Read the model definition and answer for the solid it produces. Units are mm, in the model's axes. Face numbers are marked on the shaded views. A direction names the side the tool comes from. Coordinates: 2 decimals unless noted, no trailing zeros. Loops run counter-clockwise (first coordinate to the right, second up) from the corner with the lowest first, then second, coordinate; pieces in that order, holes last. Notation, with made-up numbers: (29.5, -14) - (59.5, -14) arc R20 cw to (59.5, 22) - close; hole circle Ø7 at (26.5, 50.5). An arc over 180 degrees is marked (long way). Use one line per item in the form item = value. Start each with the question number.
1) Which of the six approach directions +Z, -Z, +X, -X, +Y, -Y give full straight-line access (tool end or side, diameter ignored) to the marked faces 1, 2, 3 and 4?
2) A cutting plane is placed at B-B (y = -1). Give the vertices of the cut face in (x, z), and give its area (3 significant figures).
3) A cutting plane is placed at D-D (x = 12.5). Give the vertices of the cut face in (y, z) (3 decimals).
4) Each of these flat-tipped pins is pushed along its axis until it touches: P1, Ø16.5, axis at x = 0, z = 0, coming from the +Y side; P2, Ø5, axis at x = 14, y = -8, coming from the +Z side; P3, Ø8, axis at x = -0.5, y = 24, coming from the -Z side; P4, Ø5, axis at x = 8, z = 12.5, coming from the +Y side. Where does it stop, or does it pass through?
5) A cutting plane is placed at A-A (x = 0). Give the vertices of the cut face in (y, z).
6) A cutting plane is placed at C-C (z = 3). Give the vertices of the cut face in (x, y).
7) The mould has two halves that part along Z. Classify the marked faces 5, 6 and 7: released by +Z, released by -Z, zero draft, split by the parting line, or undercut.
8) Consider line 1 (X direction, y = -19, z = 0); line 2 (Z direction, x = 0, y = 7); line 3 (Y direction, x = -8.5, z = 8.5). Determine where each line is inside the solid, lowest interval first.
from build123d import *

# Parameters (mm, degrees)
F0_R     = 15.24
F0_R_2   = 10.414
F1_DEPTH = 26.67
F2_DEPTH = 38.1
F4_DEPTH = 26.67
F3_R     = 10.414
F5_DEPTH = 19.05
F7_DEPTH = 4.572


with BuildPart() as f1:
    # F0 (on Front) → F1 (new body)
    with BuildSketch(Plane.XZ):
        with BuildLine():
            Line((-17.78, 10.8124097937), (-17.78, -3.556))
            ThreePointArc((-17.78, -3.556), (0, -21.336), (17.78, -3.556))
            Line((17.78, -3.556), (17.78, 10.8124097937))
            ThreePointArc((17.78, 10.8124097937), (14.6565413174, 13.9872436172), (10.9767640135, 16.4961882046))
            ThreePointArc((10.9767640135, 16.4961882046), (0, 11.8282387054), (-10.9767640135, 16.4961882046))
            ThreePointArc((-10.9767640135, 16.4961882046), (-14.6565413174, 13.9872436172), (-17.78, 10.8124097937))
        make_face()
        with Locations((0, -3.556)):
            Circle(F0_R, mode=Mode.SUBTRACT)
        with Locations((0, -3.556)):
            Circle(F0_R)
        Circle(F0_R_2, mode=Mode.SUBTRACT)
    extrude(amount=F1_DEPTH)

    # F0 (on Front) → F2 (join)
    with BuildSketch(Plane.XZ):
        with Locations((0, -3.556)):
            Circle(F0_R)
        Circle(F0_R_2, mode=Mode.SUBTRACT)
    extrude(amount=-F2_DEPTH)

    # F3 (on face) → F4 (cut)
    with BuildSketch(Plane.XZ.offset(26.67)):
        Polygon((-13.462, 14.478), (-13.462, 8.128), (-13.462, 4.064), (-10.668, 4.064), (-10.668, 12.192), (-10.668, 14.478), align=None)
    extrude(amount=-F4_DEPTH, mode=Mode.SUBTRACT)

    # F3 (on face) → F5 (cut)
    with BuildSketch(Plane.XZ.offset(26.67)):
        with BuildLine():
            Line((-15.494, 8.128), (-15.494, 0))
            ThreePointArc((-15.494, 0), (6.7794053956, -13.9321103384), (9.5613373542, 12.192))
            Line((9.5613373542, 12.192), (3.3098522596, 12.192))
            ThreePointArc((3.3098522596, 12.192), (0, 11.8282387054), (-3.3098522596, 12.192))
            Line((-3.3098522596, 12.192), (-10.668, 12.192))
            Line((-10.668, 12.192), (-10.668, 4.064))
            Line((-10.668, 4.064), (-13.462, 4.064))
            Line((-13.462, 4.064), (-13.462, 8.128))
            Line((-13.462, 8.128), (-15.494, 8.128))
        make_face()
        Circle(F3_R, mode=Mode.SUBTRACT)
    extrude(amount=-F5_DEPTH, mode=Mode.SUBTRACT)

    # F6 (on face) → F7 (cut)
    with BuildSketch(Plane(origin=(0, 0, 0), x_dir=(-1, 0, 0), z_dir=(0, 1, 0))):
        with BuildLine():
            Line((-15.24, -3.556), (-17.78, -3.556))
            ThreePointArc((-17.78, -3.556), (0, -21.336), (17.78, -3.556))
            Line((17.78, -3.556), (15.24, -3.556))
            ThreePointArc((15.24, -3.556), (0, -18.796), (-15.24, -3.556))
        make_face()
    extrude(amount=-F7_DEPTH, mode=Mode.SUBTRACT)


solid = f1.part
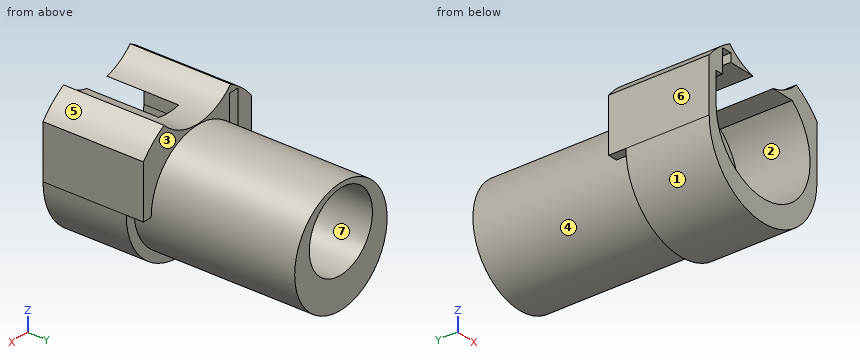
Found:
q1.face_1 = -Z, +Y, -Y
q1.face_2 = -Y
q1.face_3 = +Z, +Y
q1.face_4 = +Y
q2.outline = (-17.78, -3.56) - (-15.24, -3.56) arc R15.24 ccw to (15.24, -3.56) - (17.78, -3.56) - (17.78, 10.81) arc R22.86 ccw to (10.98, 16.5) arc R15.24 cw to (-10.98, 16.5) arc R22.86 ccw to (-17.78, 10.81) - close; hole (-13.46, 4.06) - (-10.67, 4.06) - (-10.67, 14.48) - (-13.46, 14.48) - close; hole circle Ø20.83 at (0, 0)
q2.area = 604 mm^2
q3.outline = (-26.67, -16.2) - (-4.572, -16.2) - (-4.572, -12.274) - (38.1, -12.274) - (38.1, 5.162) - (0, 5.162) - (0, 15.584) - (-26.67, 15.584) - (-26.67, 9.155) - (-7.62, 9.155) - (-7.62, -9.155) - (-26.67, -9.155) - close
q4.P1 = through
q4.P2 = 16.2
q4.P3 = -18.8
q4.P4 = 0
q5.outline = (-26.67, -21.34) - (-4.57, -21.34) - (-4.57, -18.8) - (38.1, -18.8) - (38.1, -10.41) - (-7.62, -10.41) - (-7.62, -15.49) - (-26.67, -15.49) - close; (-7.62, 10.41) - (38.1, 10.41) - (38.1, 11.68) - (0, 11.68) - (0, 11.83) - (-7.62, 11.83) - close
q6.outline = (-17.78, -26.67) - (-15.49, -26.67) - (-15.49, -7.62) - (-9.97, -7.62) - (-9.97, 38.1) - (-13.76, 38.1) - (-13.76, 0) - (-17.78, 0) - close; (9.97, -7.62) - (15.2, -7.62) - (15.2, -26.67) - (17.78, -26.67) - (17.78, 0) - (13.76, 0) - (13.76, 38.1) - (9.97, 38.1) - close
q7.face_5 = released by +Z
q7.face_6 = zero draft
q7.face_7 = undercut
q8.line_1 = -17.78 to -15.49, 15.49 to 17.78
q8.line_2 = -18.8 to -10.41, 10.41 to 11.68
q8.line_3 = -7.62 to 38.1
